Build history of the part. All positions in model axes, mm. A direction names the side the tool comes from. Give positions to 0.01 mm unless a question says otherwise; leave off trailing zeros. Loops run counter-clockwise (first coordinate to the right, second up) from the corner with the lowest first, then second, coordinate; pieces in that order, holes last. Notation, with made-up numbers: (79.5, 32) -> (99.5, 32) arc R31 cw to (99.5, 58) -> close; hole circle Ø9 at (37.5, -7.5). An arc over 180 degrees is marked (long way). One line per question, with ' | ' between items. Start each with the question number.
(1) Flat gauge pins, fed straight in: pin 1 Ø0.7 at (y, z) = (2, 0.5) entering from +X; pin 2 Ø2 at (y, z) = (5.5, 2) entering from -X; pin 3 Ø1.5 at (y, z) = (15, -1.5) entering from -X. Where does each tip first touch, or does it go through?
(2) Slice it at A-A, the plane y = 1.5. Write the cut outline in (x, z).
(3) 3-axis set-ups, long thin cutter, end or side, ignore diameter. For faces 4 (the face through (0, 19, 0)), 5 (the face through (2.44, 11.76, -0.54)), 6 (the face through (2, 1, 0)): which of +Z, -Z, +X, -X, +Y, -Y reach the whole face in a straight line?
(4) Slice it at C-C, the plane y = 7. Write the cut outline in (x, z), then the cut area to 3 significant figures.
(5) Drill centre lines: L1, parallel to X at y = 15, z = -1.5; L2, parallel to Y at x = -0.5, z = 1.5. Where is each one in solid material? Low to high. Write a range as from..to.
(6) Slice it at B-B, the plane z = 0. Write the cut outline in (x, y).
(7) Mould opens along X. For faces 1 (the face through (-3.584, 2.566, 2.285)), 2 (the face through (-1, 0, 2)), 3 (the face through (0.986, 1.479, -1.726)) say: pulls with the +X half, pulls with the -X half, needs draft (parallel to the pull), parting line crosses it, or undercut.
```python
from build123d import *

# Parameters (mm, degrees)
F2_SIZE  = 0.5
F3_R     = 0.2
F5_DEPTH = 3


with BuildPart() as f1:
    # F0 (on Right) → F1 (revolve)
    with BuildSketch(Plane.YZ):
        Polygon((0, 4.25), (0, 0), (19, 0), (19, 2.5), (5, 2.5), (5, 4.25), align=None)
    revolve(axis=Axis((0, 9.5, 0), (0, -1, 0)))

    # F2
    f2_edges = [f1.edges().sort_by_distance(p)[0] for p in [
        (0, 19, -2.5),
    ]]
    chamfer(f2_edges, length=F2_SIZE)

    # F3
    f3_edges = [f1.edges().sort_by_distance(p)[0] for p in [
        (0, 5, -2.5),
        (0, 0, -4.25),
    ]]
    fillet(f3_edges, radius=F3_R)

    # F4 (on face) → F5 (cut)
    with BuildSketch(Plane.XZ):
        Polygon((2, -1.135782), (2, 1.135782), (0, 2.3), (-2, 1.135782), (-2, -1.135782), (0, -2.3), align=None)
    extrude(amount=-F5_DEPTH, mode=Mode.SUBTRACT)


solid = f1.part
```
Final values:
1) pin 1: x = 4.25 | pin 2: x = -4.1 | pin 3: x = -2.38
2) outline: circle Ø8.5 at (0, 0); hole (-2, -1.14) -> (0, -2.3) -> (2, -1.14) -> (2, 1.14) -> (0, 2.3) -> (-2, 1.14) -> close
3) face 4: +Z, -Z, +X, -X, +Y | face 5: +Y | face 6: -Y
4) outline: circle Ø5 at (0, 0) | area: 19.6 mm2
5) L1: -2..2 | L2: 3..19
6) outline: (-4.25, 0.2) arc R0.2 ccw to (-4.05, 0) -> (-2, 0) -> (-2, 3) -> (2, 3) -> (2, 0) -> (4.05, 0) arc R0.2 ccw to (4.25, 0.2) -> (4.25, 5) -> (2.7, 5) arc R0.2 cw to (2.5, 5.2) -> (2.5, 18.5) -> (2, 19) -> (-2, 19) -> (-2.5, 18.5) -> (-2.5, 5.2) arc R0.2 cw to (-2.7, 5) -> (-4.25, 5) -> close
7) face 1: parting line crosses it | face 2: needs draft | face 3: undercut
